Check sheet for the modelled part. Datum: model origin and axes. Units: mm. A direction names the side the tool comes from. Round coordinates to 2 decimals unless told otherwise and drop trailing zeros. Order: outer loops, then holes, each group sorted by start corner. A loop starts at its lowest first (then second) coordinate and runs counter-clockwise, first axis right, second up.
(1) Depth check by flat-ended pin: pin 1 (1.2 mm diameter, centred on x = 23, y = 28, fed in from -Z); pin 2 (6 mm diameter, centred on x = 24.5, z = 5, fed in from -Y); pin 3 (6 mm diameter, centred on y = 18.5, z = 5.5, fed in from +X). Enter the tip coordinate at first touch or a pass-through.
(2) Sectioned sample at B-B, the plane x = 11. Enter the section's corners in (y, z), and give its area (3 significant figures).
(3) Tool access check on faces 1 (the cylindrical face through (14.222, 40.226, -0.423)), 2 (the flat face through (24, 28, -9)), 3 (the flat face through (24, 28, 9)), 4 (the flat face through (22, 4.5, 0)). Record the directions out of +Z, -Z, +X, -X, +Y, -Y that give a thin tool (end or side, any length) a straight path to the whole face; none if there is none.
(4) Mould release check, pull along Z, two halves, no side actions. Record for faces 5 (the flat face through (22, 3, -3.25)), 6 (the cylindrical face through (22.304, 27.768, 4.512)), 7 (the flat face through (-24, 28, 9)): released by +Z, released by -Z, zero draft, split by the parting line, or undercut.
(5) Sectioned sample at C-C, the plane y = 35. Enter the section's corners in (x, z).
(6) Sectioned sample at A-A, the plane x = -24.5. Enter the section's corners in (y, z).
(7) Sectioned sample at D-D, the plane x = -1. Enter the section's corners in (y, z), and give its area (3 significant figures).
(8) Thickness scan on probe 1 along X at (y, z) = (28.35, 5); probe 2 along Y at (x, z) = (8, -4.25); probe 3 along Z at (x, y) = (-24, 27). Record the ranges inside material, lowest first.
```python
from build123d import *

# Parameters (mm, degrees)
SKETCH1_W           = 41
SKETCH1_H           = 20
BOSS_EXTRUDE1_DEPTH = 36
BOSS_EXTRUDE2_START = -26.5
SKETCH2_W           = 55.5
SKETCH2_H           = 18
BOSS_EXTRUDE2_DEPTH = 2.5
SKETCH3_W           = 6.5
SKETCH3_H           = 3.5
BOSS_EXTRUDE3_DEPTH = 3
SKETCH4_R           = 7
BOSS_EXTRUDE4_DEPTH = 2.5
BOSS_EXTRUDE4_TAPER = 30
SKETCH5_R           = 3.25
BOSS_EXTRUDE6_DEPTH = 8
SKETCH6_R           = 6.5
BOSS_EXTRUDE7_DEPTH = 2
SKETCH9_R           = 2.25
CUT_EXTRUDE1_DEPTH  = 10


with BuildPart() as part:
    # Sketch1 → Boss-Extrude1 (new body)
    with BuildSketch(Plane(origin=(0, 0, 0), x_dir=(1, 0, 0), z_dir=(0, 1, 0))):
        Rectangle(SKETCH1_W, SKETCH1_H)
    extrude(amount=BOSS_EXTRUDE1_DEPTH)

    # Sketch2 → Boss-Extrude2 (add)
    with BuildSketch(Plane.XZ.offset(BOSS_EXTRUDE2_START)):
        Rectangle(SKETCH2_W, SKETCH2_H)
    extrude(amount=-BOSS_EXTRUDE2_DEPTH)

    # Sketch3 → Boss-Extrude3 (add)
    with BuildSketch(Plane(origin=(20.5, 0, 0), x_dir=(0, 0, -1), z_dir=(1, 0, 0))):
        with Locations((0, 2.75)):
            Rectangle(SKETCH3_W, SKETCH3_H)
    extrude(amount=BOSS_EXTRUDE3_DEPTH)

    # Sketch4 → Boss-Extrude4 (add)
    with BuildSketch(Plane(origin=(0, 36, 0), x_dir=(1, 0, 0), z_dir=(0, 1, 0))):
        with Locations((11, 0)):
            Circle(SKETCH4_R)
    extrude(amount=BOSS_EXTRUDE4_DEPTH, taper=BOSS_EXTRUDE4_TAPER)

    # Sketch5 → Boss-Extrude6 (add)
    with BuildSketch(Plane(origin=(0, 36, 0), x_dir=(1, 0, 0), z_dir=(0, 1, 0))):
        with Locations(Location((11, 0, 0), (0, 0, 270))):
            Circle(SKETCH5_R)
    extrude(amount=BOSS_EXTRUDE6_DEPTH)

    # Sketch6 → Boss-Extrude7 (add)
    with BuildSketch(Plane(origin=(0, 44, 0), x_dir=(1, 0, 0), z_dir=(0, 1, 0))):
        with Locations(Location((11, 0, 0), (0, 0, 270))):
            Circle(SKETCH6_R)
    extrude(amount=-BOSS_EXTRUDE7_DEPTH)

    # Sketch9 → Cut-Extrude1 (cut)
    with BuildSketch(Plane(origin=(0, 29, 0), x_dir=(1, 0, 0), z_dir=(0, 1, 0))):
        with Locations(Location((-24.5, 5, 0), (0, 0, 270))):
            Circle(SKETCH9_R)
        with Locations(Location((24.5, 5, 0), (0, 0, 90))):
            Circle(SKETCH9_R)
        with Locations(Location((-24.5, -5, 0), (0, 0, 90))):
            Circle(SKETCH9_R)
        with Locations(Location((24.5, -5, 0), (0, 0, 270))):
            Circle(SKETCH9_R)
    extrude(amount=-CUT_EXTRUDE1_DEPTH, mode=Mode.SUBTRACT)


solid = part.part
```
Derived:
1. pin 1: stops at z = -9
1. pin 2: stops at y = 1
1. pin 3: stops at x = 20.5
2. outline: (0, -10) - (36, -10) - (36, -7) - (38.5, -5.56) - (38.5, -3.25) - (42, -3.25) - (42, -6.5) - (44, -6.5) - (44, 6.5) - (42, 6.5) - (42, 3.25) - (38.5, 3.25) - (38.5, 5.56) - (36, 7) - (36, 10) - (0, 10) - close
2. area: 800 mm2
3. face 1: none
3. face 2: -Z, +X, +Y, -Y
3. face 3: +Z, +X, +Y, -Y
3. face 4: +Z, -Z, +X
4. face 5: released by -Z
4. face 6: undercut
4. face 7: released by +Z
5. outline: (-20.5, -10) - (20.5, -10) - (20.5, 10) - (-20.5, 10) - close
6. outline: (26.5, -9) - (29, -9) - (29, -7.25) - (26.5, -7.25) - close; (26.5, -2.75) - (29, -2.75) - (29, 2.75) - (26.5, 2.75) - close; (26.5, 7.25) - (29, 7.25) - (29, 9) - (26.5, 9) - close
7. outline: (0, -10) - (36, -10) - (36, 10) - (0, 10) - close
7. area: 720 mm2
8. probe 1: x = -27.75 to -26.75, -22.25 to 22.25, 26.75 to 27.75
8. probe 2: y = 0 to 38.5, 42 to 44
8. probe 3: z = -9 to -7.19, -2.81 to 2.81, 7.19 to 9
